Source: CAD feature listing. Evaluate the final solid. Frame: model axes, mm. Face numbers are marked on the shaded views. A direction names the side the tool comes from. Give positions to 0.01 mm unless a question says otherwise; leave off trailing zeros. Write each loop counter-clockwise with the first axis right and the second up, starting at its lowest first coordinate (ties: lowest second). Pieces come first, ordered by that corner, then holes. Notation, with made-up numbers: (49, -19) -> (55, -19) arc R25 ccw to (55, -1) -> close; hole circle Ø6 at (56, 53). An arc over 180 degrees is marked (long way). Write item = value, one per line.
Solid Edge part; units mm, degrees
sketch "Sketch1" plane through (0, 0, 0) normal (0, -1, 0) x (1, 0, 0)
  line L0 (0, 54.5) -> (0, 12.5)
  line L1 (5, 12.5) -> (0, 12.5)
  line L2 (5, 59.5) -> (5, 12.5)
  line L3 (5, 59.5) -> (-12, 59.5)
  line L4 (-12, 59.5) -> (-12, 54.5)
  line L5 (-12, 54.5) -> (0, 54.5)
  dimension "D1" = 5
  dimension "D2" = 12
  dimension "D3" = 12
revolve "RevolvedProtrusion1" add sketch "Sketch1" angle 360 about axis through (0, 0, 0) along (1, 0, 0)
sketch "Sketch2" plane through (0, 0, 0) normal (0, 1, 0) x (-1, 0, 0)
  line L0 (-5, 12.5) -> (-5, 14.5)
  line L1 (-5, 14.5) -> (-15, 14.5)
  line L2 (-15, 14.5) -> (-15, 12.5)
  line L3 (-15, 12.5) -> (-5, 12.5)
  dimension "D1" = 15
  dimension "D2" = 15
revolve "RevolvedProtrusion2" add sketch "Sketch2" angle 360 about axis through (0, 0, 0) along (1, 0, 0)
fillet "Round1" radius 2 1 edges at (5, 0, 14.5)
fillet "Round_7" radius 5 1 edges at (5, 0, -59.5)
properties material "Steel"
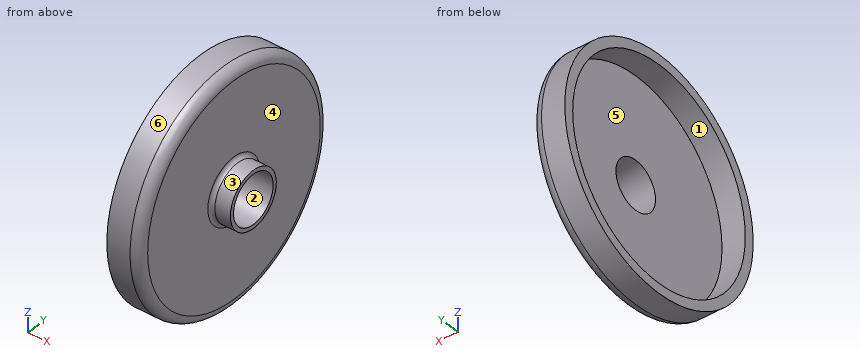
(1) Pull-direction query (Z, two-part tool) for the marked faces 4, 5 and 6; classes: pulls with the +Z half, pulls with the -Z half, needs draft (parallel to the pull), parting line crosses it, or undercut.
Values follow:
face_4 = needs draft
face_5 = undercut
face_6 = parting line crosses it
(2) Access query for the marked faces 1, 2 and 3. Directions: +Z, -Z, +X, -X, +Y, -Y. A direction counts if a zero-diameter tool reaches every point of the face in a straight line with its end or side. Return the directions, or none.
Values follow:
face_1 = -X
face_2 = +X, -X
face_3 = +X
(3) Section query C-C (x = -5). Return loops of the section in (y, z).
Values follow:
outline = circle Ø119 at (0, 0); hole circle Ø109 at (0, 0)
(4) Material intervals for line 1 (Z direction, x = 8, y = 0); line 2 (Z direction, x = -5.25, y = 0), sorted ascending.
Values follow:
line_1 = -14.5 to -12.5, 12.5 to 14.5
line_2 = -59.5 to -54.5, 54.5 to 59.5
(5) First-contact query: pin 1 (6 mm diameter, centred on x = 1.5, y = -21, fed in from -Z); pin 2 (5 mm diameter, centred on y = -8.5, z = 34, fed in from +X); pin 3 (8 mm diameter, centred on x = -8, z = -33, fed in from -Y). Flat tips, straight axial feed; report the tip coordinate or a pass-through.
Values follow:
pin_1 = -56.63
pin_2 = 5
pin_3 = -51.95
(6) Section query A-A (z = 0). Return loops of the section in (x, y).
Values follow:
outline = (-12, -59.5) -> (0, -59.5) arc R5 ccw to (5, -54.5) -> (5, -16.5) arc R2 cw to (7, -14.5) -> (15, -14.5) -> (15, -12.5) -> (0, -12.5) -> (0, -54.5) -> (-12, -54.5) -> close; (-12, 54.5) -> (0, 54.5) -> (0, 12.5) -> (15, 12.5) -> (15, 14.5) -> (7, 14.5) arc R2 cw to (5, 16.5) -> (5, 54.5) arc R5 ccw to (0, 59.5) -> (-12, 59.5) -> close
